from build123d import *

# Parameters (mm, degrees)
BOSS_EXTRUDE1_DEPTH      = 11.6
BOSS_EXTRUDE2_DEPTH      = 8
SKETCH2_R                = 7.167468034
BOSS_EXTRUDE3_DEPTH      = 1
BOSS_EXTRUDE4_START      = -1
SKETCH3_R                = 7.167468034
SKETCH3_R_2              = 5.4
BOSS_EXTRUDE4_DEPTH      = 1
FILLET1_R                = 1
WRAP1_SECTION_W          = 3
WRAP1_SECTION_H          = 4.5
WRAP1_ANGLE              = 28.285258241
WRAP1_SECTOR_2_SECTION_W = 3
WRAP1_SECTOR_2_SECTION_H = 4.5
WRAP1_SECTOR_2_ANGLE     = 28.285258241
WRAP2_START              = 1
WRAP2_DEPTH              = 4.5
SKETCH6_R                = 1
CUT_EXTRUDE1_DEPTH       = 6


# Read off the part's stored shape, not the designer's step: Wrap2
with BuildPart() as part:
    # Sketch1 → Boss-Extrude1 (new body)
    with BuildSketch(Plane(origin=(0, 0, 0), x_dir=(1, 0, 0), z_dir=(0, 1, 0))):
        with BuildLine():
            ThreePointArc((-7.167468034, 0), (0, 7.167468034), (7.167468034, 0))
            Line((7.167468034, 0), (7.9, 0))
            ThreePointArc((7.9, 0), (7.765790365, 1.45), (7.367721519, 2.850733172))
            ThreePointArc((7.367721519, 2.850733172), (0, 7.9), (-7.367721519, 2.850733172))
            ThreePointArc((-7.367721519, 2.850733172), (-7.765790365, 1.45), (-7.9, 0))
            Line((-7.9, 0), (-7.167468034, 0))
        make_face()
        with BuildLine():
            Line((7.9, 0), (7.167468034, 0))
            ThreePointArc((7.167468034, 0), (0, -7.167468034), (-7.167468034, 0))
            Line((-7.167468034, 0), (-7.9, 0))
            ThreePointArc((-7.9, 0), (-7.765790365, -1.45), (-7.367721519, -2.850733172))
            ThreePointArc((-7.367721519, -2.850733172), (0, -7.9), (7.367721519, -2.850733172))
            ThreePointArc((7.367721519, -2.850733172), (7.765790365, -1.45), (7.9, 0))
        make_face()
    extrude(amount=BOSS_EXTRUDE1_DEPTH)

    # Sketch1<3> → Boss-Extrude2 (add)
    with BuildSketch(Plane(origin=(0, 0, 0), x_dir=(1, 0, 0), z_dir=(0, 1, 0))):
        with BuildLine():
            ThreePointArc((-7.367721519, -2.850733172), (-7.765790365, -1.45), (-7.9, 0))
            Line((-7.9, 0), (-10.8, 0))
            ThreePointArc((-10.8, 0), (-9.75288861, -2.230875119), (-7.367721519, -2.850733172))
        make_face()
        with BuildLine():
            Line((-10.8, 0), (-7.9, 0))
            ThreePointArc((-7.9, 0), (-7.765790365, 1.45), (-7.367721519, 2.850733172))
            ThreePointArc((-7.367721519, 2.850733172), (-9.75288861, 2.230875119), (-10.8, 0))
        make_face()
        with BuildLine():
            ThreePointArc((7.367721519, 2.850733172), (7.765790365, 1.45), (7.9, 0))
            Line((7.9, 0), (10.8, 0))
            ThreePointArc((10.8, 0), (9.75288861, 2.230875119), (7.367721519, 2.850733172))
        make_face()
        with BuildLine():
            Line((10.8, 0), (7.9, 0))
            ThreePointArc((7.9, 0), (7.765790365, -1.45), (7.367721519, -2.850733172))
            ThreePointArc((7.367721519, -2.850733172), (9.75288861, -2.230875119), (10.8, 0))
        make_face()
    extrude(amount=BOSS_EXTRUDE2_DEPTH)

    # Sketch2 → Boss-Extrude3 (add)
    with BuildSketch(Plane(origin=(0, 0, 0), x_dir=(1, 0, 0), z_dir=(0, 1, 0))):
        with Locations(Location((0, 0, 0), (0, 0, 270))):
            Circle(SKETCH2_R)
    extrude(amount=BOSS_EXTRUDE3_DEPTH)

    # Sketch3 → Boss-Extrude4 (add)
    with BuildSketch(Plane(origin=(0, 11.6, 0), x_dir=(1, 0, 0), z_dir=(0, 1, 0)).offset(BOSS_EXTRUDE4_START)):
        with Locations(Location((0, 0, 0), (0, 0, 270))):
            Circle(SKETCH3_R)
        with Locations(Location((0, 0, 0), (0, 0, 270))):
            Circle(SKETCH3_R_2, mode=Mode.SUBTRACT)
    extrude(amount=BOSS_EXTRUDE4_DEPTH)

    # Fillet1
    fillet1_edges = [part.edges().sort_by_distance(p)[0] for p in [
        (7.9, 11.6, 0),
    ]]
    fillet(fillet1_edges, radius=FILLET1_R)

    # Wrap1 section (on wrap section) → Wrap1 (revolve, cut)
    with BuildSketch(Plane(origin=(0, 0, 0), x_dir=(-0.8056126558283049, 0, -0.5924426122159557), z_dir=(-0.5924426122159557, 0, 0.8056126558283049))):
        with Locations((6.4, -3.25)):
            Rectangle(WRAP1_SECTION_W, WRAP1_SECTION_H)
    revolve(axis=Axis((0, 0, 0), (0, -1, 0)), revolution_arc=WRAP1_ANGLE, mode=Mode.SUBTRACT)

    # Wrap1 sector 2 section (on wrap section) → Wrap1 sector 2 (revolve, cut)
    with BuildSketch(Plane(origin=(0, 0, 0), x_dir=(0.4286861079278577, 0, -0.9034534967941986), z_dir=(-0.9034534967941986, 0, -0.4286861079278577))):
        with Locations((6.4, -3.25)):
            Rectangle(WRAP1_SECTOR_2_SECTION_W, WRAP1_SECTOR_2_SECTION_H)
    revolve(axis=Axis((0, 0, 0), (0, -1, 0)), revolution_arc=WRAP1_SECTOR_2_ANGLE, mode=Mode.SUBTRACT)

    # Wrap2 outline → Wrap2 (cut)
    with BuildSketch(Plane(origin=(0, 0, 0), x_dir=(1, 0, 0), z_dir=(0, 1, 0)).offset(WRAP2_START)):
        with BuildLine():
            ThreePointArc((5.774202958, -4.246313485), (4.561660138, -5.528458629), (3.072593975, -6.475474058))
            Line((3.072593975, -6.475474058), (3.386620253, -7.137282625))
            ThreePointArc((3.386620253, -7.137282625), (5.027872453, -6.093480007), (6.364339981, -4.680296637))
            Line((6.364339981, -4.680296637), (5.774202958, -4.246313485))
        make_face()
        with BuildLine():
            Line((-3.386620253, -7.137282625), (-3.072593975, -6.475474058))
            ThreePointArc((-3.072593975, -6.475474058), (-4.561660138, -5.528458629), (-5.774202958, -4.246313485))
            Line((-5.774202958, -4.246313485), (-6.364339981, -4.680296637))
            ThreePointArc((-6.364339981, -4.680296637), (-5.027872453, -6.093480007), (-3.386620253, -7.137282625))
        make_face()
    extrude(amount=WRAP2_DEPTH, mode=Mode.SUBTRACT)

    # Sketch6 → Cut-Extrude1 (cut)
    with BuildSketch(Plane.XZ):
        with Locations(Location((-8, 0, 0), (0, 0, 270))):
            Circle(SKETCH6_R)
        with Locations(Location((8, 0, 0), (0, 0, 270))):
            Circle(SKETCH6_R)
    extrude(amount=-CUT_EXTRUDE1_DEPTH, mode=Mode.SUBTRACT)


solid = part.part
Build history of the part. All positions in model axes, mm. A direction names the side the tool comes from. Coordinates: 2 decimals unless noted, no trailing zeros. Write each loop counter-clockwise with the first axis right and the second up, starting at its lowest first coordinate (ties: lowest second). Pieces come first, ordered by that corner, then holes. Notation, with made-up numbers: (69, 76.5) -> (88, 76.5) arc R14 ccw to (88, 100.5) -> close; hole circle Ø2 at (9, 61.5). An arc over 180 degrees is marked (long way). Use CSV: the item, a comma, the result in double quotes. Start each with the question number.
Q1. Drill centre lines: probe 1 along Y at (x, z) = (-6.5, -1.5); probe 2 along Z at (x, y) = (-8, 2.05); probe 3 along Z at (x, y) = (0.25, 4). Where is each one in solid material? Low to high.
Q2. Flat gauge pins, fed straight in: pin 1 Ø2.5 at (x, z) = (10, 0) entering from +Y; pin 2 Ø2.5 at (x, z) = (-8, 0) entering from -Y; pin 3 Ø4 at (x, y) = (5, 7.5) entering from -Z; pin 4 Ø1.5 at (x, y) = (4, 6) entering from +Z. Where does each tip first touch, or does it go through?
Q3. Cut at C-C, the plane y = 9.5. List the corners of the cut face in (x, z).
Q4. Cut at D-D, the plane x = 5. State how many separate pieces and enclosed holes the cut face has, then the cut area to 3 significant figures.
Q5. Cut at A-A, the plane y = 7.5. List the corners of the cut face in (x, z), then the cut area to 3 significant figures.
Q6. Cut at B-B, the plane y = 4.5. List the corners of the cut face in (x, z).
Q7. Pull direction Z, two halves, no side cores. Call faces 5 (the flat face through (-8, 6, 0)), 6 (the flat face through (-4, 11.6, -4)): released by +Z, released by -Z, zero draft, split by the parting line, or undercut.
Q8. 3-axis set-ups, long thin cutter, end or side, ignore diameter. For faces 1 (the flat face through (0, 0, 0)), 2 (the cylindrical face through (-6.836, 6.799, -2.153)), 3 (the cylindrical face through (1.62, 11.09, 5.15)), 4 (the cylindrical face through (-9, 3, 0)): which of +Z, -Z, +X, -X, +Y, -Y reach the whole face in a straight line?
Checked values:
1,probe 1,"y = 0 to 1, 10.6 to 11.6"
1,probe 2,"z = -2.9 to -1, 1 to 2.9"
1,probe 3,"z = -7.9 to -7.16, 7.16 to 7.9"
2,pin 1,"stops at y = 8"
2,pin 2,"stops at y = 0"
2,pin 3,"stops at z = -7.31"
2,pin 4,"stops at z = 7.2"
3,outline,"circle Ø15.8 at (0, 0); hole circle Ø14.33 at (0, 0)"
4,separate pieces,"3"
4,enclosed holes,"0"
4,area,"29.8 mm²"
5,outline,"(-7.37, -2.85) arc R7.9 ccw to (7.37, -2.85) arc R2.9 ccw (long way) to (7.37, 2.85) arc R7.9 ccw to (-7.37, 2.85) arc R2.9 ccw (long way) to start; hole circle Ø14.33 at (0, 0)"
5,area,"63.2 mm²"
6,outline,"(-7.37, -2.85) arc R7.9 ccw to (-6.36, -4.68) -> (-5.77, -4.25) arc R7.17 cw to (-7.15, -0.52) arc R1 cw (long way) to (-7.15, 0.52) arc R7.17 cw to (-5.77, 4.25) -> (-6.36, 4.68) arc R7.9 ccw to (-7.37, 2.85) arc R2.9 ccw (long way) to start; (-3.39, -7.14) arc R7.9 ccw to (3.39, -7.14) -> (3.07, -6.48) arc R7.17 cw to (-3.07, -6.48) -> close; (-3.39, 7.14) -> (-3.07, 6.48) arc R7.17 cw to (3.07, 6.48) -> (3.39, 7.14) arc R7.9 ccw to start; (5.77, -4.25) -> (6.36, -4.68) arc R7.9 ccw to (7.37, -2.85) arc R2.9 ccw (long way) to (7.37, 2.85) arc R7.9 ccw to (6.36, 4.68) -> (5.77, 4.25) arc R7.17 cw to (7.15, 0.52) arc R1 cw (long way) to (7.15, -0.52) arc R7.17 cw to start"
7,face 5,"undercut"
7,face 6,"zero draft"
8,face 1,"+Z, -Z, +X, -X, -Y"
8,face 2,"none"
8,face 3,"+Y"
8,face 4,"-Y"
